For this review, take the finished solid that the model builds, in its own axes (mm). A direction names the side the tool comes from. Round coordinates to 2 decimals unless told otherwise and drop trailing zeros. Order: outer loops, then holes, each group sorted by start corner. A loop starts at its lowest first (then second) coordinate and runs counter-clockwise, first axis right, second up. Notation, with made-up numbers: (63.5, -31.5) -> (70.5, -31.5) arc R29 cw to (70.5, 2.5) -> close; hole circle Ø3 at (23, 24). An arc over 180 degrees is marked (long way). Put each result on its own line as item: value. Start each with the question number.
```python
from build123d import *

# Parameters (mm, degrees)
SKETCH1_W           = 711.2
SKETCH1_H           = 965.2
SKETCH1_W_2         = 76.2
SKETCH1_H_2         = 939.8
BOSS_EXTRUDE1_DEPTH = 50.8
SKETCH2_W           = 711.2
SKETCH2_H           = 127
BOSS_EXTRUDE2_DEPTH = 82.55
SKETCH3_W           = 711.2
SKETCH3_H           = 127
BOSS_EXTRUDE3_DEPTH = 82.55
SKETCH4_W           = 1130.3
SKETCH4_H           = 127
BOSS_EXTRUDE4_DEPTH = 82.55
SKETCH5_W           = 1130.3
SKETCH5_H           = 127
BOSS_EXTRUDE5_DEPTH = 82.55
CHAMFER1_SIZE       = 25.4


with BuildPart() as part:
    # Sketch1 → Boss-Extrude1 (new body)
    with BuildSketch(Plane(origin=(0, 0, 0), x_dir=(1, 0, 0), z_dir=(0, 1, 0))):
        Rectangle(SKETCH1_W, SKETCH1_H)
        with Locations((-304.8, 0)):
            Rectangle(SKETCH1_W_2, SKETCH1_H_2, mode=Mode.SUBTRACT)
        with Locations((304.8, 0)):
            Rectangle(SKETCH1_W_2, SKETCH1_H_2, mode=Mode.SUBTRACT)
    extrude(amount=BOSS_EXTRUDE1_DEPTH)

    # Sketch2 → Boss-Extrude2 (add)
    with BuildSketch(Plane.XY.offset(482.6)):
        with Locations((0, 88.9)):
            Rectangle(SKETCH2_W, SKETCH2_H)
    extrude(amount=BOSS_EXTRUDE2_DEPTH)

    # Sketch3 → Boss-Extrude3 (add)
    with BuildSketch(Plane(origin=(0, 0, -482.6), x_dir=(-1, 0, 0), z_dir=(0, 0, -1))):
        with Locations((0, 88.9)):
            Rectangle(SKETCH3_W, SKETCH3_H)
    extrude(amount=BOSS_EXTRUDE3_DEPTH)

    # Sketch4 → Boss-Extrude4 (add)
    with BuildSketch(Plane(origin=(355.6, 0, 0), x_dir=(0, 0, -1), z_dir=(1, 0, 0))):
        with Locations((0, 88.9)):
            Rectangle(SKETCH4_W, SKETCH4_H)
    extrude(amount=BOSS_EXTRUDE4_DEPTH)

    # Sketch5 → Boss-Extrude5 (add)
    with BuildSketch(Plane.ZY.offset(355.6)):
        with Locations((0, 88.9)):
            Rectangle(SKETCH5_W, SKETCH5_H)
    extrude(amount=BOSS_EXTRUDE5_DEPTH)

    # Chamfer1
    chamfer1_edges = [part.edges().sort_by_distance(p)[0] for p in [
        (0, 25.4, 565.15),
        (0, 152.4, 565.15),
        (0, 25.4, -565.15),
        (0, 152.4, -565.15),
        (438.15, 88.9, 565.15),
        (438.15, 25.4, 0),
        (438.15, 88.9, -565.15),
        (438.15, 152.4, 0),
        (-438.15, 88.9, -565.15),
        (-438.15, 25.4, 0),
        (-438.15, 88.9, 565.15),
        (-438.15, 152.4, 0),
    ]]
    chamfer(chamfer1_edges, length=CHAMFER1_SIZE)


solid = part.part
```
Item 1: Consider section A-A, the plane x = -318. Write out the cut boundary in (y, z).
Item 2: Consider section D-D, the plane x = -164. Write out the cut boundary in (y, z).
Item 3: For L1, parallel to X at y = 17, z = 97.5; L2, parallel to X at y = 117, z = 16; L3, parallel to X at y = 49.5, z = 64.5, list the stretches that pass through material, from the lowest coordinate up.
Item 4: Insertion check: pin 1 Ø12.5 at (y, z) = (10.5, -0.5) entering from +X; pin 2 Ø12.5 at (x, y) = (-59.5, 13) entering from +Z; pin 3 Ø12 at (x, y) = (-269.5, 47.5) entering from -Z; pin 4 Ø2 at (x, y) = (257, 44.5) entering from -Z. Each pin has a flat end and moves straight along its axis. Give the tip position at first contact, or say it passes through.
Item 5: Consider section C-C, the plane y = 37.5. Write out the cut boundary in (x, z), plus the area to 3 significant figures.
Item 6: Mouldability with a two-part tool opening along X and no side actions: class faces 1 (the face through (422.4, 134.7, -547.8)), 2 (the face through (-5, 102, 482.6)), 3 (the face through (-422.45, 42.77, 547.42)), 4 (the face through (304, 25, -469.9)) as +X half, -X half, draft (parallel to the pull), parting line (faces both ways), or undercut.
Item 7: Consider section B-B, the plane z = -159.5. Write out the cut boundary in (x, y).
Item 8: Tool access review of faces 5 (the face through (-305, 25, -469.9)), 6 (the face through (-355.6, 13, 7)), 7 (the face through (-5, 13, 482.6)), 8 (the face through (-5, 50.8, -7)): name each direction out of +Z, -Z, +X, -X, +Y, -Y from which nothing blocks a thin tool from reaching the whole face with its end or side.
Evaluation:
1. outline: (0, -482.6) -> (25.4, -482.6) -> (25.4, -539.75) -> (50.8, -565.15) -> (127, -565.15) -> (152.4, -539.75) -> (152.4, -482.6) -> (50.8, -482.6) -> (50.8, -469.9) -> (0, -469.9) -> close; (0, 469.9) -> (50.8, 469.9) -> (50.8, 482.6) -> (152.4, 482.6) -> (152.4, 539.75) -> (127, 565.15) -> (50.8, 565.15) -> (25.4, 539.75) -> (25.4, 482.6) -> (0, 482.6) -> close
2. outline: (0, -482.6) -> (25.4, -482.6) -> (25.4, -539.75) -> (50.8, -565.15) -> (127, -565.15) -> (152.4, -539.75) -> (152.4, -482.6) -> (50.8, -482.6) -> (50.8, 482.6) -> (152.4, 482.6) -> (152.4, 539.75) -> (127, 565.15) -> (50.8, 565.15) -> (25.4, 539.75) -> (25.4, 482.6) -> (0, 482.6) -> close
3. L1: x = -355.6 to -342.9, -266.7 to 266.7, 342.9 to 355.6
3. L2: x = -438.15 to -355.6, 355.6 to 438.15
3. L3: x = -436.85 to -342.9, -266.7 to 266.7, 342.9 to 436.85
4. pin 1: stops at x = 355.6
4. pin 2: stops at z = 482.6
4. pin 3: stops at z = -565.15
4. pin 4: stops at z = -559.85
5. outline: (-424.85, -539.75) -> (-412.75, -551.85) -> (412.75, -551.85) -> (424.85, -539.75) -> (424.85, 539.75) -> (412.75, 551.85) -> (-412.75, 551.85) -> (-424.85, 539.75) -> close; hole (-342.9, -469.9) -> (-266.7, -469.9) -> (-266.7, 469.9) -> (-342.9, 469.9) -> close; hole (266.7, -469.9) -> (342.9, -469.9) -> (342.9, 469.9) -> (266.7, 469.9) -> close
5. area: 794,000 mm^2
6. face 1: +X half
6. face 2: undercut
6. face 3: -X half
6. face 4: undercut
7. outline: (-438.15, 50.8) -> (-412.75, 25.4) -> (-355.6, 25.4) -> (-355.6, 0) -> (-342.9, 0) -> (-342.9, 50.8) -> (-355.6, 50.8) -> (-355.6, 152.4) -> (-412.75, 152.4) -> (-438.15, 127) -> close; (-266.7, 0) -> (266.7, 0) -> (266.7, 50.8) -> (-266.7, 50.8) -> close; (342.9, 0) -> (355.6, 0) -> (355.6, 25.4) -> (412.75, 25.4) -> (438.15, 50.8) -> (438.15, 127) -> (412.75, 152.4) -> (355.6, 152.4) -> (355.6, 50.8) -> (342.9, 50.8) -> close
8. face 5: +Y, -Y
8. face 6: +Z, -Z, -X, -Y
8. face 7: +Z, +X, -X, -Y
8. face 8: +Y
